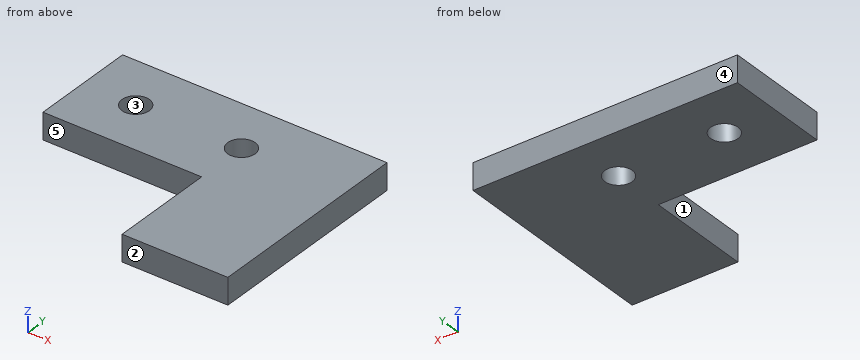
Autodesk Inventor part; units mm, degrees
ref_plane "YZ Plane" through (0, 0, 0) normal (1, 0, 0) x (0, 1, 0)
ref_plane "XZ Plane" through (0, 0, 0) normal (0, 1, 0) x (-1, 0, 0)
ref_plane "XY Plane" through (0, 0, 0) normal (0, 0, 1) x (1, 0, 0)
sketch "Sketch1" plane through (0, 0, 0) normal (0, 0, 1) x (1, 0, 0)
  circle A0 centre (0, 0) radius 5.5
  line L0 (12.6998, 0) -> (-114.3002, 0)
  line L1 (-114.3002, 0) -> (63.4998, 0)
  line L2 (63.4998, 0) -> (63.4998, -152.4)
  line L3 (63.4998, 0) -> (63.4998, 152.4)
  line L4 (63.4998, 152.4) -> (38.0998, 152.4)
  line L5 (63.4998, 152.4) -> (63.4998, 127)
  line L6 (63.4998, 127) -> (88.8998, 127)
  line L7 (88.8998, 127) -> (88.8998, 177.8)
  line L8 (88.8998, 177.8) -> (25.3998, 177.8)
  line L9 (25.3998, 177.8) -> (25.3998, 152.4)
  line L10 (25.3998, 152.4) -> (38.0998, 152.4)
  circle A1 centre (63.5, 165.1) radius 3.5 construction
  circle A2 centre (38.1, 165.1) radius 3.5 construction
  circle A3 centre (63.5, 165.1) radius 3.302
  circle A4 centre (38.1, 165.1) radius 3.302
  point P0 (0, 0)
  dimension "d0" = 127
  dimension "d1" = 177.8
  dimension "d2" = 152.4
  dimension "d3" = 152.4
  dimension "d4" = 25.4
  dimension "d5" = 25.4
  dimension "d6" = 25.4
  dimension "d7" = 50.8
  dimension "d8" = 63.5
  dimension "d11" = 6.604
  dimension "d12" = 6.604
extrude "Extrusion2" add sketch "Sketch1" along normal blind 6.35 contours L3 L4 L10 L9 L8 L7 L6
properties part number "vrRig_v08_breadboardAlignment"
Check sheet for the modelled part. Datum: model origin and axes. Units: mm. Face numbers are marked on the shaded views. A direction names the side the tool comes from. Give positions to 0.01 mm unless a question says otherwise; leave off trailing zeros. Write each loop counter-clockwise with the first axis right and the second up, starting at its lowest first coordinate (ties: lowest second). Pieces come first, ordered by that corner, then holes. Notation, with made-up numbers: (88.25, -21.5) -> (92.25, -21.5) arc R34 cw to (92.25, 14.5) -> close; hole circle Ø7 at (-18.5, 9). An arc over 180 degrees is marked (long way). One line per item, written item: value. Start each with the question number.
Item 1: Section check D-D on y = 136. Record the cut outline in (x, z).
Item 2: Draft check along X on the marked faces 1, 2 and 3. Enter one of: +X half, -X half, draft (parallel to the pull), parting line (faces both ways), or undercut.
Item 3: Gauge pin test, flat ends, axial feed: pin 1 (3 mm diameter, centred on x = 44, y = 167, fed in from -Z); pin 2 (3 mm diameter, centred on y = 142.5, z = 4.5, fed in from -X). Record the tip position at first contact, or that the pin passes through.
Item 4: Tool access check on the marked faces 4 and 5. Record the directions out of +Z, -Z, +X, -X, +Y, -Y that give a thin tool (end or side, any length) a straight path to the whole face; none if there is none.
Item 5: Section check B-B on z = 5. Record the cut outline in (x, y), then the cut area to 3 significant figures.
Item 6: Material ranges on probe 1 along X at (y, z) = (165.1, 2); probe 2 along Y at (x, z) = (38.1, 4.5); probe 3 along X at (y, z) = (166, 1.5), recorded low to high. Write a range as from..to.
Item 7: Section check C-C on y = 165.1. Record the cut outline in (x, z), then the cut area to 3 significant figures.
Item 8: Section check A-A on x = 38.1. Record the cut outline in (y, z).
Results list:
1. outline: (63.5, 0) -> (88.9, 0) -> (88.9, 6.35) -> (63.5, 6.35) -> close
2. face 1: -X half
2. face 2: draft
2. face 3: undercut
3. pin 1: z = 0
3. pin 2: x = 63.5
4. face 4: +Z, -Z, +X, -X, +Y
4. face 5: +Z, -Z, -X, -Y
5. outline: (25.4, 152.4) -> (63.5, 152.4) -> (63.5, 127) -> (88.9, 127) -> (88.9, 177.8) -> (25.4, 177.8) -> close; hole circle Ø6.6 at (38.1, 165.1); hole circle Ø6.6 at (63.5, 165.1)
5. area: 2,190 mm²
6. probe 1: 25.4..34.8, 41.4..60.2, 66.8..88.9
6. probe 2: 152.4..161.8, 168.4..177.8
6. probe 3: 25.4..34.92, 41.28..60.32, 66.68..88.9
7. outline: (25.4, 0) -> (34.8, 0) -> (34.8, 6.35) -> (25.4, 6.35) -> close; (41.4, 0) -> (60.2, 0) -> (60.2, 6.35) -> (41.4, 6.35) -> close; (66.8, 0) -> (88.9, 0) -> (88.9, 6.35) -> (66.8, 6.35) -> close
7. area: 319 mm²
8. outline: (152.4, 0) -> (161.8, 0) -> (161.8, 6.35) -> (152.4, 6.35) -> close; (168.4, 0) -> (177.8, 0) -> (177.8, 6.35) -> (168.4, 6.35) -> close
